CAD build for the part. Positions are in the model's coordinates, mm. A direction names the side the tool comes from. Round coordinates to 2 decimals unless told otherwise and drop trailing zeros. Order: outer loops, then holes, each group sorted by start corner. A loop starts at its lowest first (then second) coordinate and runs counter-clockwise, first axis right, second up. Notation, with made-up numbers: (83.25, -17.5) - (107.25, -17.5) arc R21 ccw to (107.25, -2.5) - close; hole circle Ø1 at (5.25, 18). An arc over 180 degrees is marked (long way). Use one line per item in the form item = value. Start each with the question number.
from build123d import *

# Parameters (mm, degrees)
F0_R     = 139.7
F0_R_2   = 138.43
F1_DEPTH = 76.2
F0_R_3   = 167.64
F2_DEPTH = 6.35
F3_T     = -2.54
F4_DEPTH = 3.81
F5_R     = 5.08
F7_DEPTH = 63.5


with BuildPart() as f1:
    # F0 (on Front) → F1 (new body)
    with BuildSketch(Plane.XZ):
        Circle(F0_R)
        Circle(F0_R_2, mode=Mode.SUBTRACT)
        Circle(F0_R_2)
    extrude(amount=F1_DEPTH)

    # F0 (on Front) → F2 (join)
    with BuildSketch(Plane.XZ):
        Circle(F0_R_3)
        Circle(F0_R, mode=Mode.SUBTRACT)
    extrude(amount=F2_DEPTH)

    # F3
    f3_openings = [f1.faces().sort_by_distance(p)[0] for p in [
        (0, 0, 0),
    ]]
    offset(amount=F3_T, openings=f3_openings, kind=Kind.INTERSECTION)

    # F0 (on Front) → F4 (cut)
    with BuildSketch(Plane.XZ):
        Circle(F0_R_3)
        Circle(F0_R, mode=Mode.SUBTRACT)
    extrude(amount=F4_DEPTH, mode=Mode.SUBTRACT)

    # F5
    f5_edges = [f1.edges().sort_by_distance(p)[0] for p in [
        (-139.7, -76.2, 0),
        (-139.7, -6.35, 0),
        (-137.16, -73.66, 0),
    ]]
    fillet(f5_edges, radius=F5_R)

    # F6 (on face) → F7 (cut)
    with BuildSketch(Plane.XZ.offset(76.2)):
        with BuildLine():
            Line((-139.7, -50.8), (-129.54, -50.8))
            Line((-129.54, -50.8), (-129.54, -36.6324009587))
            ThreePointArc((-129.54, -36.6324009587), (-134.62, 0), (-129.54, 36.6324009587))
            Line((-129.54, 36.6324009587), (-129.54, 50.8))
            Line((-129.54, 50.8), (-139.7, 50.8))
            Line((-139.7, 50.8), (-139.7, -50.8))
        make_face()
        with BuildLine():
            ThreePointArc((134.62, 0), (133.3439522438, -18.4914791188), (129.54, -36.6324009587))
            Line((129.54, -36.6324009587), (129.54, -50.8))
            Line((129.54, -50.8), (139.7, -50.8))
            Line((139.7, -50.8), (139.7, 50.8))
            Line((139.7, 50.8), (129.54, 50.8))
            Line((129.54, 50.8), (129.54, 36.6324009587))
            ThreePointArc((129.54, 36.6324009587), (133.3439522438, 18.4914791188), (134.62, 0))
        make_face()
        with BuildLine():
            ThreePointArc((-129.54, 36.6324009587), (-134.62, 0), (-129.54, -36.6324009587))
            Line((-129.54, -36.6324009587), (-129.54, 36.6324009587))
        make_face()
        with BuildLine():
            Line((129.54, 36.6324009587), (129.54, -36.6324009587))
            ThreePointArc((129.54, -36.6324009587), (133.3439522438, -18.4914791188), (134.62, 0))
            ThreePointArc((134.62, 0), (133.3439522438, 18.4914791188), (129.54, 36.6324009587))
        make_face()
        with BuildLine():
            Line((-50.8, 129.54), (-36.6324009587, 129.54))
            ThreePointArc((-36.6324009587, 129.54), (0, 134.62), (36.6324009587, 129.54))
            Line((36.6324009587, 129.54), (50.8, 129.54))
            Line((50.8, 129.54), (50.8, 139.7))
            Line((50.8, 139.7), (-50.8, 139.7))
            Line((-50.8, 139.7), (-50.8, 129.54))
        make_face()
        with BuildLine():
            ThreePointArc((36.6324009587, 129.54), (0, 134.62), (-36.6324009587, 129.54))
            Line((-36.6324009587, 129.54), (36.6324009587, 129.54))
        make_face()
        with BuildLine():
            Line((36.6324009587, -129.54), (-36.6324009587, -129.54))
            ThreePointArc((-36.6324009587, -129.54), (0, -134.62), (36.6324009587, -129.54))
        make_face()
        with BuildLine():
            ThreePointArc((36.6324009587, -129.54), (0, -134.62), (-36.6324009587, -129.54))
            Line((-36.6324009587, -129.54), (-50.8, -129.54))
            Line((-50.8, -129.54), (-50.8, -139.7))
            Line((-50.8, -139.7), (50.8, -139.7))
            Line((50.8, -139.7), (50.8, -129.54))
            Line((50.8, -129.54), (36.6324009587, -129.54))
        make_face()
    extrude(amount=-F7_DEPTH, mode=Mode.SUBTRACT)


solid = f1.part
(1) Slice it at B-B (y = -20). Give the cut face in (x, z), and give its area (3 significant figures).
(2) Slice it at A-A (x = 0). Give the cut face in (y, z).
(3) Which spindle directions (+Z, -Z, +X, -X, +Y, -Y) get a long thin tool onto all of the face, cutting with end or side? Do faces 1 (the flat face through (12, -75, -129.54)), 2 (the flat face through (129.54, -75, 12)), 3 (the cylindrical face through (64.46, -40.86, -123.94)). Say none if no direction does.
(4) Slice it at C-C (z = 0). Give the cut face in (x, y), and give its area (3 significant figures).
(5) Wall check: line 1 (Y direction, x = 23, z = -56.5); line 2 (X direction, y = -19, z = 97); line 3 (X direction, y = -46.5, z = 86.5). Give the ranges that are in metal, low to high. Write a range as [from, to].
(6) Flat gauge pins, fed straight in: P1, Ø1, axis at y = -58, z = -115.5, coming from the +X side; P2, Ø6, axis at x = 47.5, y = -52, coming from the +Z side; P3, Ø5, axis at x = -135, z = -22, coming from the -Y side; P4, Ø3, axis at x = 3, z = 135.5, coming from the -Y side. Where does each tip first touch, or does it go through?
Results list:
q1.outline = (-130.14, -50.8) arc R139.7 ccw to (-50.8, -130.14) - (-50.8, -129.54) - (-45.08, -129.54) arc R137.16 cw to (-129.54, -45.08) - (-129.54, -50.8) - close; (-130.14, 50.8) - (-129.54, 50.8) - (-129.54, 45.08) arc R137.16 cw to (-45.08, 129.54) - (-50.8, 129.54) - (-50.8, 130.14) arc R139.7 ccw to start; (45.08, -129.54) - (50.8, -129.54) - (50.8, -130.14) arc R139.7 ccw to (130.14, -50.8) - (129.54, -50.8) - (129.54, -45.08) arc R137.16 cw to start; (45.08, 129.54) arc R137.16 cw to (129.54, 45.08) - (129.54, 50.8) - (130.14, 50.8) arc R139.7 ccw to (50.8, 130.14) - (50.8, 129.54) - close
q1.area = 1,200 mm²
q2.outline = (-76.2, -129.54) - (-73.66, -129.54) - (-73.66, 129.54) - (-76.2, 129.54) - close; (-12.7, -139.7) - (-11.43, -139.7) arc R5.08 cw to (-6.35, -144.78) - (-6.35, -167.64) - (-3.81, -167.64) - (-3.81, -137.16) - (-12.7, -137.16) - close; (-12.7, 137.16) - (-3.81, 137.16) - (-3.81, 167.64) - (-6.35, 167.64) - (-6.35, 144.78) arc R5.08 cw to (-11.43, 139.7) - (-12.7, 139.7) - close
q3.face_1 = -Z, -Y
q3.face_2 = +X, -Y
q3.face_3 = -Y
q4.outline = (-167.64, -6.35) - (-144.78, -6.35) arc R5.08 cw to (-139.7, -11.43) - (-139.7, -12.7) - (-137.16, -12.7) - (-137.16, -3.81) - (-167.64, -3.81) - close; (-129.54, -76.2) - (129.54, -76.2) - (129.54, -73.66) - (-129.54, -73.66) - close; (137.16, -12.7) - (139.7, -12.7) - (139.7, -11.43) arc R5.08 cw to (144.78, -6.35) - (167.64, -6.35) - (167.64, -3.81) - (137.16, -3.81) - close
q4.area = 856 mm²
q5.line_1 = [-76.2, -73.66]
q5.line_2 = [-100.53, -96.97], [96.97, 100.53]
q5.line_3 = [-109.7, -106.45], [106.45, 109.7]
q6.P1 = 79.32
q6.P2 = 129.54
q6.P3 = -12.7
q6.P4 = through
